from build123d import *

# Parameters (mm, degrees)
SKETCH1_W           = 43
SKETCH1_H           = 43
SKETCH1_R           = 2.25
SKETCH1_R_2         = 1.65
BOSS_EXTRUDE1_DEPTH = 0.5
SKETCH2_R           = 6
CUT_EXTRUDE1_DEPTH  = 1
FILLET1_R           = 2.5
CHAMFER1_SIZE       = 0.1
SKETCH3_R           = 1.5
CUT_EXTRUDE2_DEPTH  = 31.42203149
SKETCH4_R           = 16
SKETCH4_R_2         = 6
SKETCH4_R_3         = 1.5
BOSS_EXTRUDE2_DEPTH = 1


with BuildPart() as part:
    # Sketch1 → Boss-Extrude1 (new, symmetric)
    with BuildSketch(Plane.XY):
        Rectangle(SKETCH1_W, SKETCH1_H)
        with Locations((-17.68, 17.68)):
            Circle(SKETCH1_R, mode=Mode.SUBTRACT)
        with Locations((17.68, -17.68)):
            Circle(SKETCH1_R, mode=Mode.SUBTRACT)
        with Locations((17.68, 17.68)):
            Circle(SKETCH1_R_2, mode=Mode.SUBTRACT)
        with Locations((-17.68, -17.68)):
            Circle(SKETCH1_R_2, mode=Mode.SUBTRACT)
    extrude(amount=BOSS_EXTRUDE1_DEPTH, both=True)

    # Sketch2 → Cut-Extrude1 (cut)
    with BuildSketch(Plane.XY.offset(0.5)):
        Circle(SKETCH2_R)
    extrude(amount=-CUT_EXTRUDE1_DEPTH, mode=Mode.SUBTRACT)

    # Fillet1
    fillet1_edges = [part.edges().sort_by_distance(p)[0] for p in [
        (21.5, -21.5, 0),
        (-21.5, -21.5, 0),
        (-21.5, 21.5, 0),
        (21.5, 21.5, 0),
    ]]
    fillet(fillet1_edges, radius=FILLET1_R)

    # Chamfer1
    chamfer1_edges = [part.edges().sort_by_distance(p)[0] for p in [
        (0, -21.5, -0.5),
        (0, -21.5, 0.5),
        (21.5, 0, -0.5),
        (-21.5, 0, -0.5),
        (0, 21.5, -0.5),
        (-20.767766953, 20.767766953, -0.5),
        (20.767766953, 20.767766953, -0.5),
        (20.767766953, -20.767766953, -0.5),
        (-20.767766953, -20.767766953, -0.5),
        (-21.5, 0, 0.5),
        (21.5, 0, 0.5),
        (0, 21.5, 0.5),
        (-20.767766953, 20.767766953, 0.5),
        (20.767766953, 20.767766953, 0.5),
        (20.767766953, -20.767766953, 0.5),
        (-20.767766953, -20.767766953, 0.5),
    ]]
    chamfer(chamfer1_edges, length=CHAMFER1_SIZE)

    # Sketch3 → Cut-Extrude2 (cut, through all)
    with BuildSketch(Plane.XY.offset(0.5)):
        with Locations((-9.42, 7.43)):
            Circle(SKETCH3_R)
        with Locations((11.15, 4.45)):
            Circle(SKETCH3_R)
        with Locations((-1.72, -11.85)):
            Circle(SKETCH3_R)
    extrude(amount=-CUT_EXTRUDE2_DEPTH, mode=Mode.SUBTRACT)

    # Sketch4 → Boss-Extrude2 (add)
    with BuildSketch(Plane(origin=(0, 0, -0.5), x_dir=(-1, 0, 0), z_dir=(0, 0, -1))):
        Circle(SKETCH4_R)
        with Locations(Location((0, 0, 0), (0, 0, 180))):
            Circle(SKETCH4_R_2, mode=Mode.SUBTRACT)
        with Locations(Location((-11.15, 4.45, 0), (0, 0, 180))):
            Circle(SKETCH4_R_3, mode=Mode.SUBTRACT)
        with Locations(Location((9.42, 7.43, 0), (0, 0, 180))):
            Circle(SKETCH4_R_3, mode=Mode.SUBTRACT)
        with Locations(Location((1.72, -11.85, 0), (0, 0, 180))):
            Circle(SKETCH4_R_3, mode=Mode.SUBTRACT)
    extrude(amount=BOSS_EXTRUDE2_DEPTH)


solid = part.part
The model under review builds one solid part; all positions refer to its coordinate system, in mm. A direction names the side the tool comes from. Give positions to 0.01 mm unless a question says otherwise; leave off trailing zeros. Order: outer loops, then holes, each group sorted by start corner. A loop starts at its lowest first (then second) coordinate and runs counter-clockwise, first axis right, second up. Notation, with made-up numbers: M 54.25,42 L 76.25,42 A16 cw 76.25,69 Z; hole C 18.5,0.25 d7. An arc over 180 degrees is marked long. Answer in a Markdown table with one row per item. Add a question column.
1. To check wall thickness, follow line 1 along Y through (x, z) = (-17.68, -0.1); line 2 along Y through (x, z) = (-2.5, -1.1); line 3 along Z through (x, y) = (18, 0.5). State the ranges of each line that lie inside material, in increasing order.
2. Mouldability with a two-part tool opening along X and no side actions: class faces 1 (the cylindrical face through (20.748, 20.787, -0.006)), 2 (the flat face through (-5, 5, 0.5)), 3 (the cylindrical face through (-19.33, -17.61, -0.01)) as released by +X, released by -X, zero draft, split by the parting line, or undercut.
3. Add section C-C on x = -9.42. State the section outline as (y, z) points, plus the area to 3 significant figures.
4. For pin 1 Ø5 at (x, y) = (17.68, -17.68) entering from -Z; pin 2 Ø1.8 at (x, y) = (-1.72, -11.85) entering from -Z, all flat-tipped, find the tip position at first contact; note any pin that passes through.
5. Machinability: for faces 4 (the cylindrical face through (-8.73, 8.76, -0.49)), 5 (the flat face through (-15, 10, -0.5)), which of the approach directions +Z, -Z, +X, -X, +Y, -Y give a long, thin tool a straight path to every point of the face, cutting with its end or side? Answer none if there is none.
6. Add section D-D on y = -14. State the section outline as (x, z) points.
7. Add section B-B on y = 7.43. State the section outline as (x, z) points, plus the area to 3 significant figures.
8. Add section A-A on y = 17.68. State the section outline as (x, z) points.
The answers:
| question | item | result |
|---|---|---|
| 1 | line 1 | -21.5 to -19.33, -16.03 to 15.43, 19.93 to 21.5 |
| 1 | line 2 | -15.8 to -13.13, -10.57 to -5.45, 5.45 to 15.8 |
| 1 | line 3 | -0.5 to 0.5 |
| 2 | face 1 | released by +X |
| 2 | face 2 | zero draft |
| 2 | face 3 | undercut |
| 3 | outline | M -21.5,-0.4 L -21.4,-0.5 L -12.93,-0.5 L -12.93,-1.5 L 5.93,-1.5 L 5.93,0.5 L -21.4,0.5 L -21.5,0.4 Z; M 8.93,-1.5 L 12.93,-1.5 L 12.93,-0.5 L 21.4,-0.5 L 21.5,-0.4 L 21.5,0.4 L 21.4,0.5 L 8.93,0.5 Z |
| 3 | area | 62.8 mm2 |
| 4 | pin 1 | z = -0.5 |
| 4 | pin 2 | through |
| 5 | face 4 | +Z, -Z |
| 5 | face 5 | -Z |
| 6 | outline | M -21.5,-0.4 L -21.4,-0.5 L -7.75,-0.5 L -7.75,-1.5 L 7.75,-1.5 L 7.75,-0.5 L 21.4,-0.5 L 21.5,-0.4 L 21.5,0.4 L 21.4,0.5 L -21.4,0.5 L -21.5,0.4 Z |
| 7 | outline | M -21.5,-0.4 L -21.4,-0.5 L -14.17,-0.5 L -14.17,-1.5 L -10.92,-1.5 L -10.92,0.5 L -21.4,0.5 L -21.5,0.4 Z; M -7.92,-1.5 L 14.17,-1.5 L 14.17,-0.5 L 21.4,-0.5 L 21.5,-0.4 L 21.5,0.4 L 21.4,0.5 L -7.92,0.5 Z |
| 7 | area | 65.3 mm2 |
| 8 | outline | M -21.5,-0.4 L -21.4,-0.5 L -19.93,-0.5 L -19.93,0.5 L -21.4,0.5 L -21.5,0.4 Z; M -15.43,-0.5 L 16.03,-0.5 L 16.03,0.5 L -15.43,0.5 Z; M 19.33,-0.5 L 21.4,-0.5 L 21.5,-0.4 L 21.5,0.4 L 21.4,0.5 L 19.33,0.5 Z |
